Read the model definition and answer for the solid it produces. Units are mm, in the model's axes. A direction names the side the tool comes from. Give positions to 0.01 mm unless a question says otherwise; leave off trailing zeros. Order: outer loops, then holes, each group sorted by start corner. A loop starts at its lowest first (then second) coordinate and runs counter-clockwise, first axis right, second up. Notation, with made-up numbers: (12, 42) - (65, 42) arc R7 cw to (65, 48) - close; hole circle Ø3 at (-28.5, -15). An arc over 180 degrees is marked (long way). Return JSON: item names as keys, results as strings.
```python
from build123d import *

# Parameters (mm, degrees)
SKETCH1_W           = 200
SKETCH1_H           = 200
SKETCH1_W_2         = 190
SKETCH1_H_2         = 190
BOSS_EXTRUDE1_DEPTH = 200
SKETCH2_W           = 200
SKETCH2_H           = 200
BOSS_EXTRUDE2_DEPTH = 5
SKETCH3_R           = 2.5
CUT_EXTRUDE1_DEPTH  = 6


with BuildPart() as part:
    # Sketch1 → Boss-Extrude1 (new body)
    with BuildSketch(Plane.XY):
        Rectangle(SKETCH1_W, SKETCH1_H)
        Rectangle(SKETCH1_W_2, SKETCH1_H_2, mode=Mode.SUBTRACT)
    extrude(amount=BOSS_EXTRUDE1_DEPTH)

    # Sketch2 → Boss-Extrude2 (add)
    with BuildSketch(Plane.XY.offset(200)):
        Rectangle(SKETCH2_W, SKETCH2_H)
    extrude(amount=BOSS_EXTRUDE2_DEPTH)

    # Sketch3 → Cut-Extrude1 (cut)
    with BuildSketch(Plane.XZ.offset(100)):
        with Locations((13, 5)):
            Circle(SKETCH3_R)
        with Locations((-13, 5)):
            Circle(SKETCH3_R)
    extrude(amount=-CUT_EXTRUDE1_DEPTH, mode=Mode.SUBTRACT)


solid = part.part
```
Q1. Given pin 1 (8 mm diameter, centred on x = 13, z = 5, fed in from -Y); pin 2 (1 mm diameter, centred on x = 41, y = 42, fed in from -Z), each flat-ended and moving along its own axis, determine where each tip first touches the part or whether it passes through.
Values:
{"pin 1": "stops at y = -100", "pin 2": "stops at z = 200"}
Q2. For faces 4 (the flat face through (100, -1, 101)), 5 (the flat face through (-95, -1, 99)), determine the directions among +Z, -Z, +X, -X, +Y, -Y from which every point of the face is accessible in a straight line to the end or side of a thin tool.
Values:
{"face 4": "+Z, -Z, +X, +Y, -Y", "face 5": "-Z"}
Q3. Determine the mould class of faces 1 (the flat face through (-1, -100, 101)), 2 (the flat face through (-1, 1, 200)), 3 (the flat face through (-1, 1, 205)) for opening direction Y: released by +Y, released by -Y, zero draft, split by the parting line, or undercut.
Values:
{"face 1": "released by -Y", "face 2": "undercut", "face 3": "zero draft"}
Q4. A cutting plane is placed at A-A (z = 133). Write down the section's boundary in (x, y).
Values:
{"outline": "(-100, -100) - (100, -100) - (100, 100) - (-100, 100) - close; hole (-95, -95) - (95, -95) - (95, 95) - (-95, 95) - close"}
Q5. Consider L1, parallel to X at y = 40, z = 82.5; L2, parallel to Z at x = 13, y = -97. Determine where each line is inside the solid, lowest interval first.
Values:
{"L1": "x = -100 to -95, 95 to 100", "L2": "z = 0 to 2.5, 7.5 to 205"}
Q6. A cutting plane is placed at B-B (y = 11.5). Write down the section's boundary in (x, z).
Values:
{"outline": "(-100, 0) - (-95, 0) - (-95, 200) - (95, 200) - (95, 0) - (100, 0) - (100, 205) - (-100, 205) - close"}
